Geometry check sheet. Reference: the model listing, model coordinates, mm. A direction names the side the tool comes from. Round coordinates to 2 decimals unless told otherwise and drop trailing zeros. Write each loop counter-clockwise with the first axis right and the second up, starting at its lowest first coordinate (ties: lowest second). Pieces come first, ordered by that corner, then holes. Notation, with made-up numbers: (12, 29.25) -> (53, 29.25) arc R20 ccw to (53, 64.25) -> close; hole circle Ø1 at (-26.5, 74.25). An arc over 180 degrees is marked (long way). Use a Markdown table: item, result.
```python
from build123d import *

# Parameters (mm, degrees)
SKETCH2_W           = 101.6
SKETCH2_H           = 50.8
BOSS_EXTRUDE1_DEPTH = 3
FILLET1_R           = 25.4
SKETCH4_W           = 25.4
SKETCH4_H           = 3
CUT_EXTRUDE1_DEPTH  = 3


with BuildPart() as part:
    # Sketch2 → Boss-Extrude1 (new body)
    with BuildSketch(Plane(origin=(0, 0, 0), x_dir=(0, 0, -1), z_dir=(1, 0, 0))):
        with Locations((50.8, 25.4)):
            Rectangle(SKETCH2_W, SKETCH2_H)
    extrude(amount=BOSS_EXTRUDE1_DEPTH)

    # Fillet1
    fillet1_edges = [part.edges().sort_by_distance(p)[0] for p in [
        (1.5, 50.8, 0),
        (1.5, 50.8, -101.6),
    ]]
    fillet(fillet1_edges, radius=FILLET1_R)

    # Sketch4 → Cut-Extrude1 (cut)
    with BuildSketch(Plane(origin=(3, 0, 0), x_dir=(0, 0, -1), z_dir=(1, 0, 0))):
        with Locations((12.7, 1.5)):
            Rectangle(SKETCH4_W, SKETCH4_H)
        with Locations((88.9, 1.5)):
            Rectangle(SKETCH4_W, SKETCH4_H)
    extrude(amount=-CUT_EXTRUDE1_DEPTH, mode=Mode.SUBTRACT)


solid = part.part
```
(1) Section check A-A on x = 1.8. Record the cut outline in (y, z), plus the area to 3 significant figures.
A:
| item | result |
|---|---|
| outline | (0, -76.2) -> (3, -76.2) -> (3, -101.6) -> (25.4, -101.6) arc R25.4 ccw to (50.8, -76.2) -> (50.8, -25.4) arc R25.4 ccw to (25.4, 0) -> (3, 0) -> (3, -25.4) -> (0, -25.4) -> close |
| area | 4,730 mm2 |
(2) Thickness scan on line 1 (Y direction, x = 1.7, z = -25); line 2 (Y direction, x = 1.9, z = -20.5); line 3 (Z direction, x = 2.25, y = 34). Record the ranges inside material, lowest first.
A:
| item | result |
|---|---|
| line 1 | y = 3 to 50.8 |
| line 2 | y = 3 to 50.32 |
| line 3 | z = -100.1 to -1.5 |
(3) Section check C-C on y = 36.5. Record the cut outline in (x, z), plus the area to 3 significant figures.
A:
| item | result |
|---|---|
| outline | (0, -99.05) -> (3, -99.05) -> (3, -2.55) -> (0, -2.55) -> close |
| area | 289 mm2 |
(4) Gauge pin test, flat ends, axial feed: pin 1 Ø1 at (x, y) = (1, 45.5) entering from +Z; pin 2 Ø1.5 at (x, z) = (2, -8.5) entering from -Y; pin 3 Ø1 at (x, y) = (2, 37.5) entering from +Z. Record the tip position at first contact, or that the pin passes through.
A:
| item | result |
|---|---|
| pin 1 | stops at z = -9.24 |
| pin 2 | stops at y = 3 |
| pin 3 | stops at z = -2.8 |
(5) Access from +Z, -Z, +X, -X, +Y, -Y to the whole of each face (thin tool, end or side, straight path). Record for faces 1 (the face through (3, 26, -50)), 2 (the face through (2, 1, -76.2)), 3 (the face through (2, 1, -25.4)).
A:
| item | result |
|---|---|
| face 1 | +Z, -Z, +X, +Y, -Y |
| face 2 | -Z, +X, -X, -Y |
| face 3 | +Z, +X, -X, -Y |
(6) Section check B-B on z = -7. Record the cut outline in (x, y), plus the area to 3 significant figures.
A:
| item | result |
|---|---|
| outline | (0, 3) -> (3, 3) -> (3, 42.91) -> (0, 42.91) -> close |
| area | 120 mm2 |
